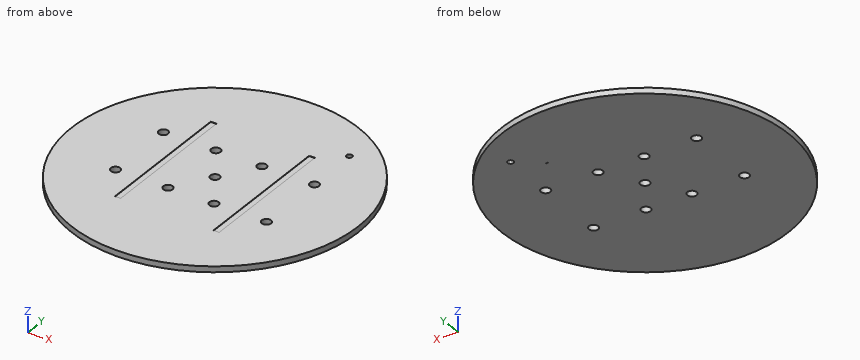
from build123d import *

# Parameters (mm, degrees)
F0_W     = 3.2
F0_H     = 80
F0_R     = 79.7
F0_R_2   = 2.6
F1_DEPTH = 3.2
F2_DEPTH = 3
F4_D     = 3.2
F4_DEPTH = 3.2


with BuildPart() as f1:
    # F0 (on Top) → F1 (new body)
    with BuildSketch(Plane.XY):
        with Locations((-27.4, 0)):
            Rectangle(F0_W, F0_H)
        Polygon((25.8, 40), (25.8, -40), (29, -40), (29, 39.927304), align=None)
        Circle(F0_R)
        with Locations((-42, -20)):
            Circle(F0_R_2, mode=Mode.SUBTRACT)
        with Locations((-12.8, -20)):
            Circle(F0_R_2, mode=Mode.SUBTRACT)
        with Locations((12.8, -20)):
            Circle(F0_R_2, mode=Mode.SUBTRACT)
        with Locations((42, -20)):
            Circle(F0_R_2, mode=Mode.SUBTRACT)
        with Locations((-42, 20)):
            Circle(F0_R_2, mode=Mode.SUBTRACT)
        with Locations((-27.4, 0)):
            Rectangle(F0_W, F0_H, mode=Mode.SUBTRACT)
        with Locations((-12.8, 20)):
            Circle(F0_R_2, mode=Mode.SUBTRACT)
        Circle(F0_R_2, mode=Mode.SUBTRACT)
        Polygon((29, -40), (25.8, -40), (25.8, 40), (29, 40), (29, 39.927304), align=None, mode=Mode.SUBTRACT)
        with Locations((12.8, 20)):
            Circle(F0_R_2, mode=Mode.SUBTRACT)
        with Locations((42, 20)):
            Circle(F0_R_2, mode=Mode.SUBTRACT)
    extrude(amount=F1_DEPTH)

    # F0 (on Top) → F2 (join)
    with BuildSketch(Plane.XY):
        with Locations((-27.4, 0)):
            Rectangle(F0_W, F0_H)
        Polygon((25.8, 40), (25.8, -40), (29, -40), (29, 39.927304), align=None)
    extrude(amount=F2_DEPTH)

    # F4
    with Locations(Plane.XY.offset(3.2)):
        with Locations((41.473566, 50.049408)):
            Hole(F4_D / 2, depth=F4_DEPTH)


solid = f1.part
The model under review builds one solid part; all positions refer to its coordinate system, in mm. Round coordinates to 2 decimals unless told otherwise and drop trailing zeros. Write each loop counter-clockwise with the first axis right and the second up, starting at its lowest first coordinate (ties: lowest second). Pieces come first, ordered by that corner, then holes. Notation, with made-up numbers: (-16.5, -10) - (-11.5, -10) arc R20 ccw to (-11.5, 0) - close; hole circle Ø9 at (-16, 76). An arc over 180 degrees is marked (long way). One line per item, written item: value. Start each with the question number.
1. Clearance check with flat-ended pins moving along their axes: P1, Ø1.5, axis at x = -5.5, z = 1, coming from the +Y side; P2, Ø3, axis at x = -42, y = -20, coming from the -Z side; P3, Ø1.6, axis at x = 28, z = 1.5, coming from the -Y side; P4, Ø1, axis at x = -27.5, y = -19, coming from the +Z side. State where each tip first meets the part, or that it passes through.
2. Consider section D-D on y = -20. Write out the cut boundary in (x, z), and give its area (3 significant figures).
3. To check wall thickness, follow L1, parallel to Y at x = 12.8, z = 1.6; L2, parallel to Y at x = -44, z = 1.1; L3, parallel to Y at x = 46.5, z = 2.45. State the ranges of each line that lie inside material, in increasing order. Write a range as from..to.
4. Consider section C-C on z = 1.7. State how many separate pieces and enclosed holes the cut face has, and give its area (3 significant figures).
5. Consider section B-B on x = 0. Write out the cut boundary in (y, z).
6. Consider section A-A on y = 0. Write out the cut boundary in (x, z), and give its area (3 significant figures).
Checks:
1. P1: stops at y = 79.56
1. P2: passes through
1. P3: stops at y = -74.91
1. P4: stops at z = 3
2. outline: (-77.15, 0) - (-44.6, 0) - (-44.6, 3.2) - (-77.15, 3.2) - close; (-39.4, 0) - (-15.4, 0) - (-15.4, 3.2) - (-25.8, 3.2) - (-25.8, 3) - (-29, 3) - (-29, 3.2) - (-39.4, 3.2) - close; (-10.2, 0) - (10.2, 0) - (10.2, 3.2) - (-10.2, 3.2) - close; (15.4, 0) - (39.4, 0) - (39.4, 3.2) - (29, 3.2) - (29, 3) - (25.8, 3) - (25.8, 3.2) - (15.4, 3.2) - close; (44.6, 0) - (77.15, 0) - (77.15, 3.2) - (44.6, 3.2) - close
2. area: 426 mm^2
3. L1: y = -78.67..-22.6, -17.4..17.4, 22.6..78.67
3. L2: y = -66.45..-21.66, -18.34..18.34, 21.66..66.45
3. L3: y = -64.73..64.73
4. separate pieces: 1
4. enclosed holes: 11
4. area: 19,800 mm^2
5. outline: (-79.7, 0) - (-2.6, 0) - (-2.6, 3.2) - (-79.7, 3.2) - close; (2.6, 0) - (79.7, 0) - (79.7, 3.2) - (2.6, 3.2) - close
6. outline: (-79.7, 0) - (-2.6, 0) - (-2.6, 3.2) - (-25.8, 3.2) - (-25.8, 3) - (-29, 3) - (-29, 3.2) - (-79.7, 3.2) - close; (2.6, 0) - (79.7, 0) - (79.7, 3.2) - (29, 3.2) - (29, 3) - (25.8, 3) - (25.8, 3.2) - (2.6, 3.2) - close
6. area: 492 mm^2
